Geometry: final body of the model. Coordinates: model frame, mm. Round coordinates to 2 decimals unless told otherwise and drop trailing zeros. Write each loop counter-clockwise with the first axis right and the second up, starting at its lowest first coordinate (ties: lowest second). Pieces come first, ordered by that corner, then holes. Notation, with made-up numbers: M 13,6.25 L 48,6.25 A23 ccw 48,17.25 Z; hole C 64.25,61.5 d5. An arc over 180 degrees is marked long. Use one line per item in the form item = value. Start each with the question number.
Item 1: Section query C-C (x = -8.5). Return loops of the section in (y, z).
Item 2: Section query A-A (y = -0.85). Return loops of the section in (x, z).
Item 3: Ray query, probe 1 along X at (y, z) = (-1.45, -69); probe 2 along Z at (x, y) = (0, -2.35); probe 3 along X at (y, z) = (-0.7, -61). Return the intervals inside material, ascending.
Item 4: Section query B-B (x = 66.5). Return loops of the section in (y, z), and give its area (3 significant figures).
Item 5: Pin query (flat end, axial travel): pin 1 Ø1.5 at (y, z) = (-1, -15) entering from -X; pin 2 Ø3.5 at (x, z) = (0, -62.08) entering from -Y. Return the tip coordinate at first contact, or that it passes through.
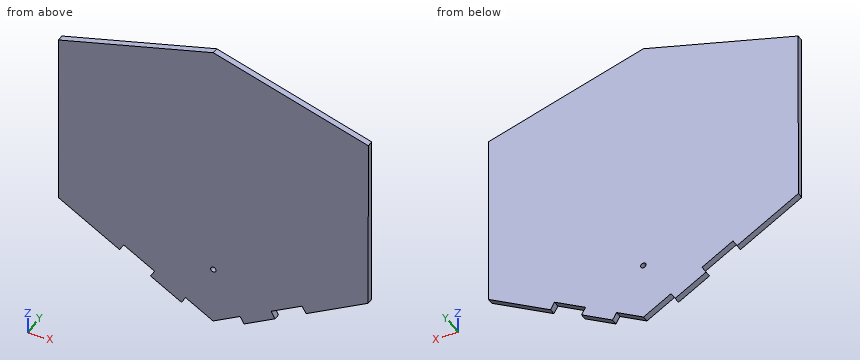
from build123d import *

# Parameters (mm, degrees)
F1_DEPTH = 3.5
F2_R     = 1.5
F3_DEPTH = 25


# Not quite as in the source:
# - a feature names something its author has since deleted; it is built from what else it names


with BuildPart() as f1:
    # F0 (on Front) → F1 (new body)
    with BuildSketch(Plane.XZ):
        Polygon((0, 75.4606574774), (-86.5353767039, 50.1161508768), (-86.6695481512, -49.8837591133), (-0.1341714472, -99.9999099901), (86.5353767039, -50.1161508768), (86.6695481512, 49.8837591133), align=None)
    extrude(amount=F1_DEPTH)

    # F2 (on face) → F3 (cut)
    with BuildSketch(Plane.XZ.offset(3.5)):
        Polygon((0.1341714472, 99.9999099901), (-17.199738183, 90.0231581674), (-14.9549690229, 86.1230285006), (0.1271996943, 94.8037622444), (-2.1236443549, 96.1073174408), align=None)
        Polygon((17.4386577754, 89.9781792171), (0.1341714472, 99.9999099901), (2.3789406073, 96.0997803233), (0.1271996943, 94.8037622444), (15.1834309859, 86.0840872654), align=None)
        Polygon((2.3789406073, 96.0997803233), (0.1341714472, 99.9999099901), (-2.1236443549, 96.1073174408), (0.1271996943, 94.8037622444), align=None)
        Polygon((-50.1288800257, -65.8258142354), (-52.3961295985, -69.7328876509), (-35.0856874223, -79.7580676974), (-32.8304606328, -75.8639757457), align=None)
        Polygon((-15.5233852921, -85.8872059211), (-17.7786120815, -89.7812978727), (-0.4715367407, -99.8045280481), (-0.3587329239, -99.6097501051), (-2.3789406073, -96.0997803233), (-0.1271996943, -94.8037622444), align=None)
        Polygon((-0.3587329239, -99.6097501051), (-0.4715367407, -99.8045280481), (-0.1341714472, -99.9999099901), align=None)
        Polygon((14.9549690229, -86.1230285006), (-0.1271996943, -94.8037622444), (1.7836900487, -95.9104360964), (-0.3587329239, -99.6097501051), (-0.1341714472, -99.9999099901), (17.199738183, -90.0231581674), align=None)
        Polygon((1.7836900487, -95.9104360964), (-0.1271996943, -94.8037622444), (-2.3789406073, -96.0997803233), (-0.3587329239, -99.6097501051), align=None)
        Polygon((34.5336478132, -80.0464063448), (51.8675574435, -70.0696545221), (49.6227882834, -66.1695248553), (32.2888786531, -76.146276678), align=None)
        with Locations((0, -62.0760797054)):
            Circle(F2_R)
    extrude(amount=-F3_DEPTH, mode=Mode.SUBTRACT)


solid = f1.part
Working result:
q1.outline = M -3.5,-89.95 L 0,-89.95 L 0,72.97 L -3.5,72.97 Z
q2.outline = M -86.67,-49.88 L -52.4,-69.73 L -50.13,-65.83 L -32.83,-75.86 L -35.09,-79.76 L -17.78,-89.78 L -15.52,-85.89 L -0.13,-94.8 L 14.95,-86.12 L 17.2,-90.02 L 34.53,-80.05 L 32.29,-76.15 L 49.62,-66.17 L 51.87,-70.07 L 86.54,-50.12 L 86.67,49.88 L 0,75.46 L -86.54,50.12 Z; hole C 0,-62.08 d3
q3.probe_1 = -53.66 to -51.97, -44.66 to 44.71, 51.25 to 53.73
q3.probe_2 = -94.73 to -63.58, -60.58 to 75.46
q3.probe_3 = -67.48 to -1.05, 1.05 to 67.63
q4.outline = M -3.5,-61.65 L 0,-61.65 L 0,55.84 L -3.5,55.84 Z
q4.area = 411 mm²
q5.pin_1 = -86.62
q5.pin_2 = -3.5
